The listing builds one solid part. Answer for the finished solid, in the listing's coordinates (mm). A direction names the side the tool comes from. Round coordinates to 2 decimals unless told otherwise and drop trailing zeros. Write each loop counter-clockwise with the first axis right and the second up, starting at its lowest first coordinate (ties: lowest second). Pieces come first, ordered by that corner, then holes.
(1) A cutting plane is placed at B-B, the plane z = -3. Give the vertices of the cut face in (x, y), and give its area (3 significant figures).
(2) Each of these flat-tipped pins is pushed along its axis until it touches: pin 1 Ø0.8 at (x, y) = (-4, 0.5) entering from +Z; pin 2 Ø0.9 at (y, z) = (-0.5, -3) entering from +X. Where does it stop, or does it pass through?
(3) For faces 1 (the face through (0, 4.85, -2)), 2 (the face through (4, -1.5, -2)), 3 (the face through (-4, 1.5, -2)), determine the directions among +Z, -Z, +X, -X, +Y, -Y from which every point of the face is accessible in a straight line to the end or side of a thin tool.
(4) The mould has two halves that part along Y. Classify faces 4 (the face through (0, -1, 0)), 5 (the face through (0, -6.25, -2)), 6 (the face through (4, 1.5, -2)), 7 (the face through (-4, -1.5, -2)): +Y half, -Y half, draft (parallel to the pull), parting line (faces both ways), or undercut.
(5) A cutting plane is placed at C-C, the plane z = -2.1. Give the vertices of the cut face in (x, y), and give its area (3 significant figures).
(6) A cutting plane is placed at A-A, the plane x = 4. Give the vertices of the cut face in (y, z).
(7) Find the intervals of material crossed by probe 1 along Y at (x, z) = (4.25, -1.95); probe 2 along X at (y, z) = (-0.25, -2.75), in increasing order.
from build123d import *

# Parameters (mm, degrees)
SKETCH006_W     = 9.5
SKETCH006_H     = 11.1
PAD004_DEPTH    = 3.5
SKETCH013_W     = 3
SKETCH013_H     = 0.65
POCKET005_DEPTH = 1
SKETCH014_W     = 9.5
SKETCH014_H     = 11.1
PAD007_DEPTH    = 0.5
FILLET007_R     = 0.5
SKETCH019_W     = 3
SKETCH019_H     = 0.65
POCKET006_DEPTH = 1
SKETCH020_W     = 3
SKETCH020_H     = 1.8
POCKET007_DEPTH = 0.3
SKETCH021_W     = 3
SKETCH021_H     = 1.8
POCKET008_DEPTH = 0.3


with BuildPart() as part:
    # Sketch006 → Pad004 (new body)
    with BuildSketch(Plane.XY):
        with Locations((0, -0.7)):
            Rectangle(SKETCH006_W, SKETCH006_H)
    extrude(amount=-PAD004_DEPTH)

    # Sketch013 (on Face4 of Pad004) → Pocket005 (cut)
    with BuildSketch(Plane.YZ.offset(4.75)):
        with Locations((0, -2.075)):
            Rectangle(SKETCH013_W, SKETCH013_H)
    extrude(amount=-POCKET005_DEPTH, mode=Mode.SUBTRACT)

    # Sketch014 (on Face5 of Pocket005) → Pad007 (join)
    with BuildSketch(Plane(origin=(0, 0, -3.5), x_dir=(-1, 0, 0), z_dir=(0, 0, -1))):
        with Locations((0, -0.7)):
            Rectangle(SKETCH014_W, SKETCH014_H)
    extrude(amount=PAD007_DEPTH)

    # Fillet007
    fillet007_edges = [part.edges().sort_by_distance(p)[0] for p in [
        (4.75, -6.25, -3.75),
        (-4.75, -6.25, -3.75),
        (4.75, 4.85, -3.75),
        (-4.75, 4.85, -3.75),
    ]]
    fillet(fillet007_edges, radius=FILLET007_R)

    # Sketch019 (on Face7 of Fillet007) → Pocket006 (cut)
    with BuildSketch(Plane(origin=(-4.75, 0, 0), x_dir=(0, -1, 0), z_dir=(-1, 0, 0))):
        with Locations((0, -2.075)):
            Rectangle(SKETCH019_W, SKETCH019_H)
    extrude(amount=-POCKET006_DEPTH, mode=Mode.SUBTRACT)

    # Sketch020 (on Face6 of Pocket006) → Pocket007 (cut)
    with BuildSketch(Plane.YZ.offset(4.75)):
        with Locations((0, -2.6)):
            Rectangle(SKETCH020_W, SKETCH020_H)
    extrude(amount=-POCKET007_DEPTH, mode=Mode.SUBTRACT)

    # Sketch021 (on Face7 of Pocket007) → Pocket008 (cut)
    with BuildSketch(Plane(origin=(-4.75, 0, 0), x_dir=(0, -1, 0), z_dir=(-1, 0, 0))):
        with Locations((0, -2.6)):
            Rectangle(SKETCH021_W, SKETCH021_H)
    extrude(amount=-POCKET008_DEPTH, mode=Mode.SUBTRACT)


solid = part.part
Solutions:
1. outline: (-4.75, -5.75) arc R0.5 ccw to (-4.25, -6.25) - (4.25, -6.25) arc R0.5 ccw to (4.75, -5.75) - (4.75, -1.5) - (4.45, -1.5) - (4.45, 1.5) - (4.75, 1.5) - (4.75, 4.35) arc R0.5 ccw to (4.25, 4.85) - (-4.25, 4.85) arc R0.5 ccw to (-4.75, 4.35) - (-4.75, 1.5) - (-4.45, 1.5) - (-4.45, -1.5) - (-4.75, -1.5) - close
1. area: 103 mm2
2. pin 1: stops at z = 0
2. pin 2: stops at x = 4.45
3. face 1: +Z, -Z, +X, -X, +Y
3. face 2: +X
3. face 3: -X
4. face 4: draft
4. face 5: -Y half
4. face 6: undercut
4. face 7: undercut
5. outline: (-4.75, -5.75) arc R0.5 ccw to (-4.25, -6.25) - (4.25, -6.25) arc R0.5 ccw to (4.75, -5.75) - (4.75, -1.5) - (3.75, -1.5) - (3.75, 1.5) - (4.75, 1.5) - (4.75, 4.35) arc R0.5 ccw to (4.25, 4.85) - (-4.25, 4.85) arc R0.5 ccw to (-4.75, 4.35) - (-4.75, 1.5) - (-3.75, 1.5) - (-3.75, -1.5) - (-4.75, -1.5) - close
5. area: 99.2 mm2
6. outline: (-6.25, -4) - (4.85, -4) - (4.85, 0) - (-6.25, 0) - close; hole (-1.5, -2.4) - (1.5, -2.4) - (1.5, -1.75) - (-1.5, -1.75) - close
7. probe 1: y = -6.25 to -1.5, 1.5 to 4.85
7. probe 2: x = -4.45 to 4.45
